For this review, take the finished solid that the model builds, in its own axes (mm). A direction names the side the tool comes from. Give positions to 0.01 mm unless a question says otherwise; leave off trailing zeros. Write each loop counter-clockwise with the first axis right and the second up, starting at its lowest first coordinate (ties: lowest second). Pieces come first, ordered by that corner, then holes.
Q1. Insertion check: P1, Ø2, axis at x = 5.5, y = 4, coming from the +Z side. The pin has a flat end and moves straight along its axis. Give the tip position at first contact, or say it passes through.
Q2. Mouldability with a two-part tool opening along X and no side actions: class faces 6 (the cylindrical face through (4.579, 3.204, 3.845)), 7 (the flat face through (3.5, 3.3, 11)), 8 (the flat face through (0, 3, 5)) as released by +X, released by -X, zero draft, split by the parting line, or undercut.
Q3. We need section C-C (y = 3.75). Write out the cut boundary in (x, z).
Q4. We need section D-D (x = 19). Write out the cut boundary in (y, z), then the cut area to 3 significant figures.
Q5. For line 1 (X direction, y = 4, z = 3.5); line 2 (Z direction, x = 5.5, y = 2.5); line 3 (X direction, y = 6, z = 2.25), list the stretches that pass through material, from the lowest coordinate up.
Q6. We need section A-A (x = 5.5). Write out the cut boundary in (y, z).
Q7. Machinability: for faces 1 (the flat face through (3.5, 4.75, 10.5)), 2 (the flat face through (3.5, 1.75, 10.5)), 3 (the flat face through (4, 3.3, 10.5)), 4 (the flat face through (21, 3, 5)), 5 (the flat face through (3, 3.2, 10.5)), which of the approach directions +Z, -Z, +X, -X, +Y, -Y give a long, thin tool a straight path to every point of the face, cutting with its end or side? Answer none if there is none.
Q8. We need section B-B (z = 3). Write out the cut boundary in (x, y).
Autodesk Inventor part; units mm, degrees
ref_plane "YZ Plane" through (0, 0, 0) normal (1, 0, 0) x (0, 1, 0)
ref_plane "XZ Plane" through (0, 0, 0) normal (0, 1, 0) x (-1, 0, 0)
ref_plane "XY Plane" through (0, 0, 0) normal (0, 0, 1) x (1, 0, 0)
sketch "Sketch1" plane through (0, 0, 0) normal (0, 0, 1) x (1, 0, 0)
  line L0 (0, 0) -> (21, 0)
  line L1 (21, 0) -> (21, 6.5)
  line L2 (21, 6.5) -> (0, 6.5)
  line L3 (0, 6.5) -> (0, 0)
  dimension "d0" = 21
  dimension "d1" = 6.5
extrude "Extrusion1" add sketch "Sketch1" along normal blind 10
sketch "Sketch2" plane through (0, 0, 10) normal (0, 0, 1) x (1, 0, 0)
  line L0 (3, 4.75) -> (4, 4.75)
  line L1 (4, 4.75) -> (4, 1.75)
  line L2 (4, 1.75) -> (3, 1.75)
  line L3 (3, 1.75) -> (3, 4.75)
  line L4 (0, 6.5) -> (0, 0)
  point P0 (3, 3.25)
  point P1 (0, 3.25)
  dimension "d4" = 1
  dimension "d5" = 3
  dimension "d6" = 3
extrude "Extrusion2" add sketch "Sketch2" along normal blind 1
sketch "Sketch3" plane through (0, 0, 0) normal (0, -1, 0) x (1, 0, 0)
  circle A0 centre (5.5, 3) radius 1.25
  circle A1 centre (15.5, 3) radius 1.25
  line L0 (5.5, 3) -> (15.5, 3) construction
  line L1 (0, 0) -> (21, 0) construction
  point P0 (10.5, 3)
  point P1 (10.5, 0)
  dimension "d9" = 2.5
  dimension "d10" = 2.5
  dimension "d11" = 3
  dimension "d12" = 10
extrude "Extrusion3" cut sketch "Sketch3" against normal through all
properties part number "relay"
Computed:
1. P1: stops at z = 10
2. face 6: undercut
2. face 7: zero draft
2. face 8: released by -X
3. outline: (0, 0) - (21, 0) - (21, 10) - (4, 10) - (4, 11) - (3, 11) - (3, 10) - (0, 10) - close; hole circle Ø2.5 at (5.5, 3); hole circle Ø2.5 at (15.5, 3)
4. outline: (0, 0) - (6.5, 0) - (6.5, 10) - (0, 10) - close
4. area: 65.0 mm2
5. line 1: x = 0 to 4.35, 6.65 to 14.35, 16.65 to 21
5. line 2: z = 0 to 1.75, 4.25 to 10
5. line 3: x = 0 to 4.5, 6.5 to 14.5, 16.5 to 21
6. outline: (0, 0) - (6.5, 0) - (6.5, 1.75) - (0, 1.75) - close; (0, 4.25) - (6.5, 4.25) - (6.5, 10) - (0, 10) - close
7. face 1: +Z, +X, -X, +Y
7. face 2: +Z, +X, -X, -Y
7. face 3: +Z, +X, +Y, -Y
7. face 4: +Z, -Z, +X, +Y, -Y
7. face 5: +Z, -X, +Y, -Y
8. outline: (0, 0) - (4.25, 0) - (4.25, 6.5) - (0, 6.5) - close; (6.75, 0) - (14.25, 0) - (14.25, 6.5) - (6.75, 6.5) - close; (16.75, 0) - (21, 0) - (21, 6.5) - (16.75, 6.5) - close
